from build123d import *

# Parameters (mm, degrees)
SKETCH1_R           = 12.7
SKETCH1_R_2         = 3.2639
SKETCH1_R_3         = 4.19989
BOSS_EXTRUDE1_DEPTH = 3.175


with BuildPart() as part:
    # Sketch1 → Boss-Extrude1 (new, symmetric)
    # profile 1 of 4: a face of its own
    with BuildSketch(Plane(origin=(0, 0, 0), x_dir=(-0.9735629333039062, 0, 0.22841894601082008), z_dir=(-0.22841894601082008, 1.7517633279464725e-15, -0.9735629333039062))):
        Circle(SKETCH1_R)
        Circle(SKETCH1_R_2, mode=Mode.SUBTRACT)
    # profile 2 of 4: a face of its own
    with BuildSketch(Plane(origin=(0, 0, 0), x_dir=(-0.9735629333039062, 0, 0.22841894601082008), z_dir=(-0.22841894601082008, 1.7517633279464725e-15, -0.9735629333039062))):
        with BuildLine():
            ThreePointArc((-2.817127899, -12.383609748), (-12.383609748, 2.817127899), (2.817127899, 12.383609748))
            Line((2.817127899, 12.383609748), (-302.209540417, 81.773646649))
            ThreePointArc((-302.209540417, 81.773646649), (-295.100250928, 77.311920379), (-292.326668316, 69.390036901))
            ThreePointArc((-292.326668316, 69.390036901), (-314.006924437, 60.40978078), (-305.026668316, 82.090036901))
            Line((-305.026668316, 82.090036901), (-473.718412785, 82.090036901))
            ThreePointArc((-473.718412785, 82.090036901), (-464.738156664, 78.370293022), (-461.018412785, 69.390036901))
            ThreePointArc((-461.018412785, 69.390036901), (-464.738156664, 60.40978078), (-473.718412785, 56.690036901))
            Line((-473.718412785, 56.690036901), (-307.87932985, 56.690036901))
            ThreePointArc((-307.87932985, 56.690036901), (-306.461910329, 56.610691476), (-305.06220195, 56.373646649))
            Line((-305.06220195, 56.373646649), (-2.817127899, -12.383609748))
        make_face()
    # profile 3 of 4: a face of its own
    with BuildSketch(Plane(origin=(0, 0, 0), x_dir=(-0.9735629333039062, 0, 0.22841894601082008), z_dir=(-0.22841894601082008, 1.7517633279464725e-15, -0.9735629333039062))):
        with Locations((-473.718412785, 69.390036901)):
            Circle(SKETCH1_R)
        with Locations((-473.718412785, 69.390036901)):
            Circle(SKETCH1_R_3, mode=Mode.SUBTRACT)
    # profile 4 of 4: a face of its own
    with BuildSketch(Plane(origin=(0, 0, 0), x_dir=(-0.9735629333039062, 0, 0.22841894601082008), z_dir=(-0.22841894601082008, 1.7517633279464725e-15, -0.9735629333039062))):
        with Locations((-305.026668316, 69.390036901)):
            Circle(SKETCH1_R)
        with Locations((-305.026668316, 69.390036901)):
            Circle(SKETCH1_R_2, mode=Mode.SUBTRACT)
    extrude(amount=BOSS_EXTRUDE1_DEPTH, both=True)


solid = part.part
Verification items for the finished model (mm, model axes). Coordinates: 2 decimals unless noted, no trailing zeros. Loops run counter-clockwise (first coordinate to the right, second up) from the corner with the lowest first, then second, coordinate; pieces in that order, holes last. Notation, with made-up numbers: M -9.75,65 L 13.25,65 A25 ccw 13.25,102 Z; hole C 84,47.25 d5. An arc over 180 degrees is marked long. One line per item, written item: value.
1. Gauge pin test, flat ends, axial feed: P1, Ø6, axis at x = 151.5, y = 50, coming from the +Z side; P2, Ø12.5, axis at x = 374.5, z = -92, coming from the -Y side; P3, Ø6, axis at x = 336, y = 63, coming from the -Z side. Record the tip position at first contact, or that the pin passes through.
Answers follow:
P1: z = -31.81
P2: y = 56.69
P3: z = -82.8
2. Section check B-B on z = -51.5. Record the cut outline in (x, y).
Answers follow:
outline: M 205.6,35.19 L 233.4,41.34 L 233.4,67.39 L 205.6,61.24 Z
3. Section check A-A on y = 51. Record the cut outline in (x, z).
Answers follow:
outline: M 161.8,-41.22 L 273.27,-67.38 L 274.73,-61.2 L 163.25,-35.04 Z
4. Material ranges on line 1 along Z through (x, y) = (434.5, 65.5); line 2 along Z through (x, y) = (256, 64.5); line 3 along Y through (x, z) = (213, -47), recorded low to high. Write a range as from..to.
Answers follow:
line 1: -105.2..-98.68
line 2: -63.32..-56.8
line 3: 36.59..62.64
